Check sheet for the drawn part. Datum: minimum x, y, z corner. Units: mm. A direction names the side the tool comes from. Round coordinates to 2 decimals unless told otherwise and drop trailing zeros. Write each loop counter-clockwise with the first axis right and the second up, starting at its lowest first coordinate (ties: lowest second). Pieces come first, ordered by that corner, then holes.
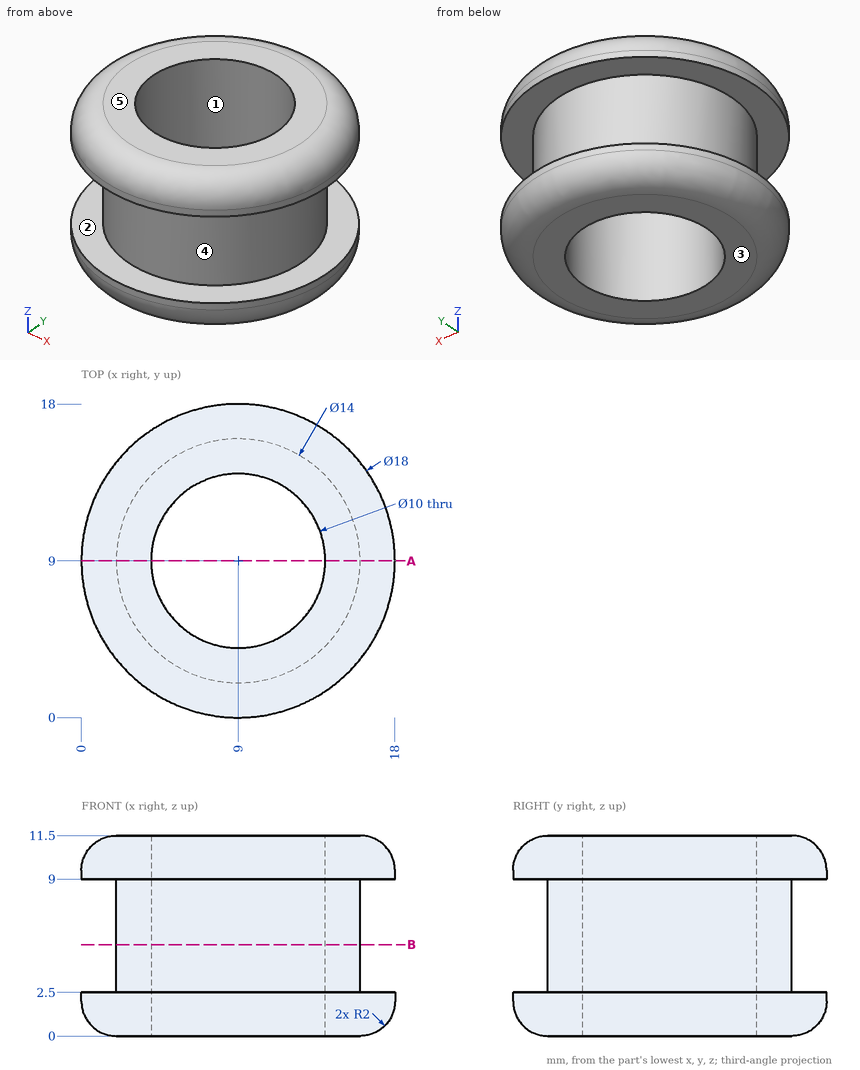
Q1. Sectioned sample at B-B (z = 5.25). Enter the section's corners in (x, y).
Recorded:
outline: circle Ø14 at (9, 9); hole circle Ø10 at (9, 9)
Q2. Depth check by flat-ended pin: P1, Ø5, axis at y = 5.5, z = 10, coming from the -X side; P2, Ø1.5, axis at x = 3.5, z = 2, coming from the +Y side; P3, Ø2, axis at y = 3.5, z = 9, coming from the +X side. Enter the tip coordinate at first touch or a pass-through.
Recorded:
P1: stops at x = 0.06
P2: stops at y = 16.64
P3: stops at x = 16.79
Q3. Material ranges on line 1 along X through (y, z) = (9, 6.25); line 2 along Y through (x, z) = (9.25, 8.5); line 3 along Y through (x, z) = (9, 9.25), recorded low to high.
Recorded:
line 1: x = 2 to 4, 14 to 16
line 2: y = 2 to 4.01, 13.99 to 16
line 3: y = 0 to 4, 14 to 18
Q4. Sectioned sample at A-A (y = 9). Enter the section's corners in (x, z).
Recorded:
outline: (0, 2) arc R2 ccw to (2, 0) - (4, 0) - (4, 11.5) - (2, 11.5) arc R2 ccw to (0, 9.5) - (0, 9) - (2, 9) - (2, 2.5) - (0, 2.5) - close; (14, 0) - (16, 0) arc R2 ccw to (18, 2) - (18, 2.5) - (16, 2.5) - (16, 9) - (18, 9) - (18, 9.5) arc R2 ccw to (16, 11.5) - (14, 11.5) - close
Q5. Tool access check on the marked faces 1 and 2. Record the directions out of +Z, -Z, +X, -X, +Y, -Y that give a thin tool (end or side, any length) a straight path to the whole face; none if there is none.
Recorded:
face 1: +Z, -Z
face 2: none
Q6. Release check for a two-part mould opening along Z. For the marked faces 3, 4 and 5 record: released by +Z, released by -Z, zero draft, split by the parting line, or undercut.
Recorded:
face 3: released by -Z
face 4: undercut
face 5: released by +Z
